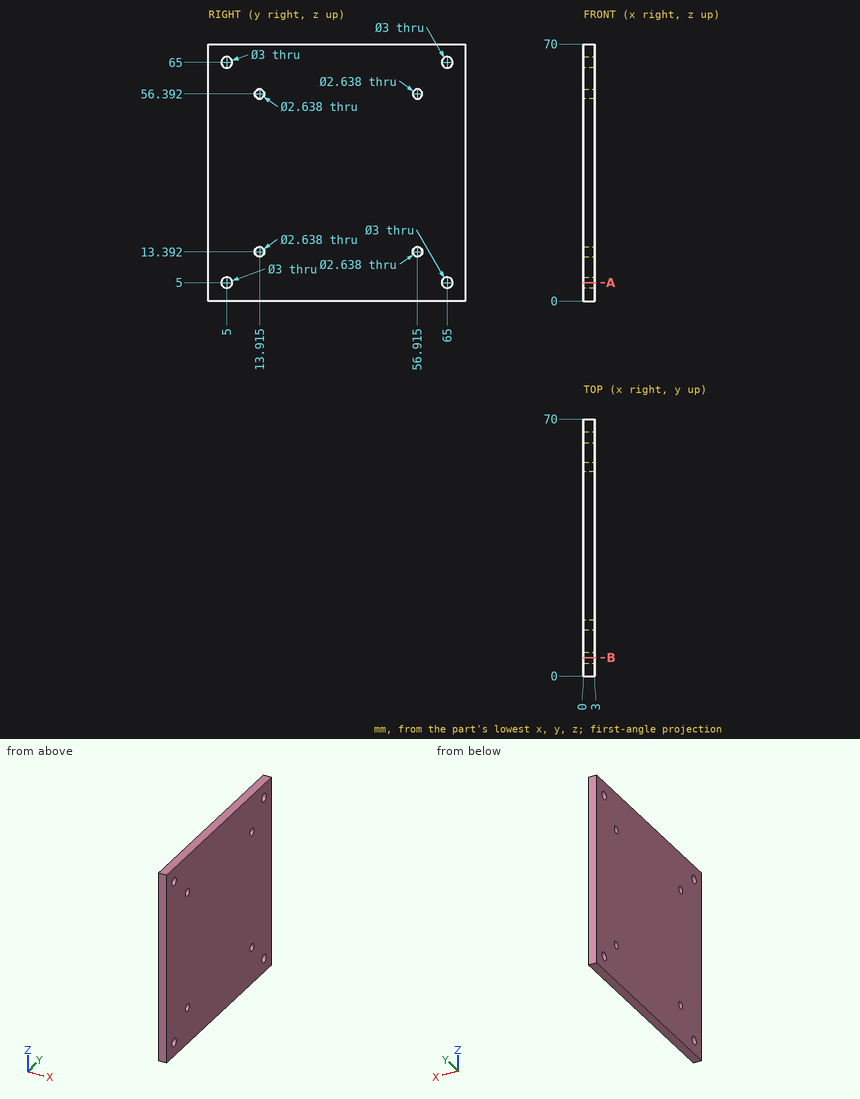
Part print with two shaded views. Sizes in mm from the minimum x, y, z corner. Round coordinates to 2 decimals unless told otherwise and drop trailing zeros. Write each loop counter-clockwise with the first axis right and the second up, starting at its lowest first coordinate (ties: lowest second). Pieces come first, ordered by that corner, then holes. Notation, with made-up numbers: M -13,8 L 40,8 A12 cw 40,29 Z; hole C 86,10.5 d3. An arc over 180 degrees is marked long. Put each result on its own line as item: value. Start each with the question number.
1) Drill centre lines: probe 1 along Y at (x, z) = (0.9, 5); probe 2 along Z at (x, y) = (2.4, 14). Where is each one in solid material? Low to high. Write a range as [from, to].
2) Saw through at A-A, the plane z = 5. Write the cut outline in (x, y).
Resolved:
1. probe 1: [0, 3.5], [6.5, 63.5], [66.5, 70]
1. probe 2: [0, 12.08], [14.71, 55.08], [57.71, 70]
2. outline: M 0,0 L 3,0 L 3,3.5 L 0,3.5 Z; M 0,6.5 L 3,6.5 L 3,63.5 L 0,63.5 Z; M 0,66.5 L 3,66.5 L 3,70 L 0,70 Z
